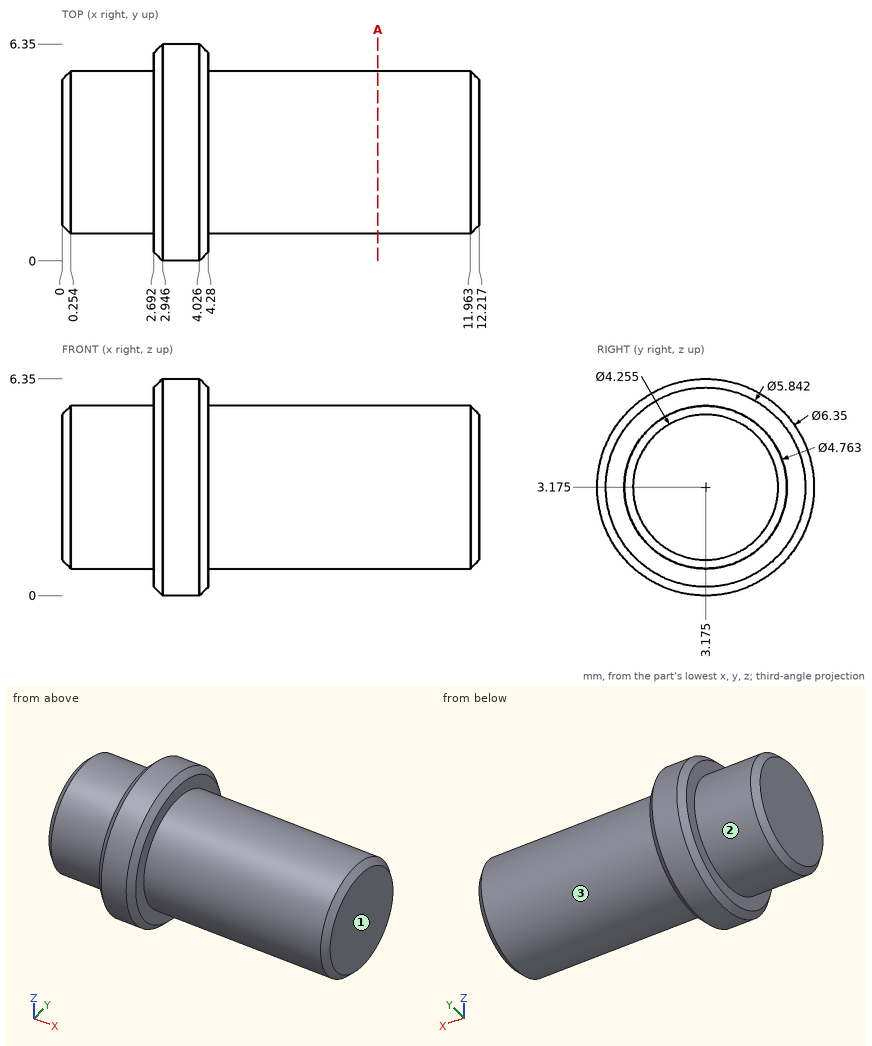
Answer from the drawing. Dimensions are ordinates in mm from the lowest x, y and z of the part. A direction names the side the tool comes from. Round coordinates to 2 decimals unless told otherwise and drop trailing zeros. Order: outer loops, then holes, each group sorted by start corner. A loop starts at its lowest first (then second) coordinate and runs counter-clockwise, first axis right, second up.
1) The part is cut by section A-A on x = 9.25. Write down the section's boundary in (y, z) (1 decimal).
2) Straight lines are drawn through the part: L1, parallel to X at y = 0.75, z = 4; L2, parallel to Y at x = 3.75, z = 5 (1 decimal); L3, parallel to Y at x = 1, z = 1.25 (1 decimal). For each, find the intervals that lie inside material, in ascending order.
3) Flat-ended cylindrical pins translate along their axes: pin 1 (1.5 mm diameter, centred on x = 2, z = 3, fed in from -Y); pin 2 (1 mm diameter, centred on x = 8, z = 3.5, fed in from +Y); pin 3 (1 mm diameter, centred on y = 1, z = 5, fed in from -X). Find the tip coordinate at first contact, or state that the pin passes through.
4) For the marked faces 1, 2 and 3, determine the directions among +Z, -Z, +X, -X, +Y, -Y from which every point of the face is accessible in a straight line to the end or side of a thin tool.
Resolved:
1. outline: circle Ø4.8 at (3.2, 3.2)
2. L1: x = 2.69 to 4.28
2. L2: y = 0.6 to 5.8
2. L3: y = 1.8 to 4.6
3. pin 1: stops at y = 0.2
3. pin 2: stops at y = 5.56
3. pin 3: stops at x = 0.21
4. face 1: +Z, -Z, +X, +Y, -Y
4. face 2: -X
4. face 3: +X
